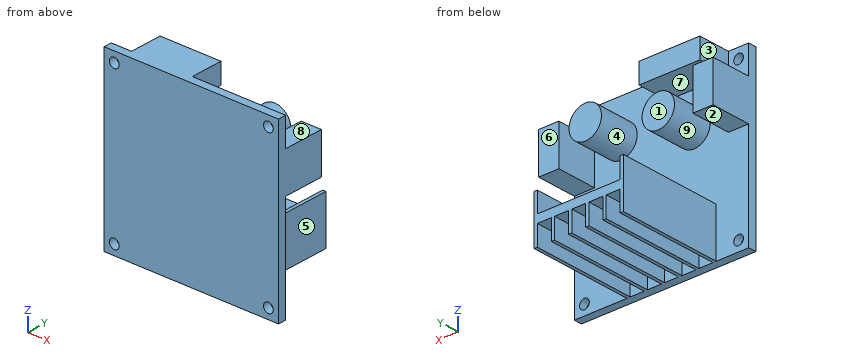
from build123d import *

# Parameters (mm, degrees)
SKETCH_1_W          = 43
SKETCH_1_H          = 43
EXTRUDE_1_DEPTH     = 2
SKETCH_2_W          = 15
SKETCH_2_H          = 5
EXTRUDE_2_DEPTH     = 10
SKETCH_3_W          = 5
SKETCH_3_H          = 10
EXTRUDE_3_DEPTH     = 10
SKETCH_4_W          = 5
SKETCH_4_H          = 10
EXTRUDE_4_DEPTH     = 10
SKETCH_5_R          = 4
EXTRUDE_5_DEPTH     = 10
SKETCH_6_R          = 4
EXTRUDE_6_DEPTH     = 10
SKETCH_7_W          = 22
SKETCH_7_H          = 12
EXTRUDE_7_DEPTH     = 26
SKETCH_8_W          = 3.44
SKETCH_8_H          = 26
SKETCH_8_H_2        = 26.05521278
CUT_EXTRUDE_1_DEPTH = 5
SKETCH_11_W         = 20.4
SKETCH_11_H         = 26
CUT_EXTRUDE_2_DEPTH = 5
SKETCH_12_W         = 20.4
SKETCH_12_H         = 7.82225214
EXTRUDE_8_DEPTH     = 5
SKETCH_13_W         = 20.4
SKETCH_13_H         = 5.214716639
EXTRUDE_9_DEPTH     = 2
SKETCH_14_R         = 1.2
CUT_EXTRUDE_3_DEPTH = 2


with BuildPart() as part:
    # 草图1 → 凸台-拉伸1 (new body)
    with BuildSketch(Plane(origin=(0, 0, 0), x_dir=(1, 0, 0), z_dir=(0, 1, 0))):
        Rectangle(SKETCH_1_W, SKETCH_1_H)
    extrude(amount=EXTRUDE_1_DEPTH)

    # 草图2 → 凸台-拉伸2 (add)
    with BuildSketch(Plane(origin=(0, 0, 0), x_dir=(1, 0, 0), z_dir=(0, 1, 0))):
        with Locations((-9, -19)):
            Rectangle(SKETCH_2_W, SKETCH_2_H)
    extrude(amount=EXTRUDE_2_DEPTH)

    # 草图3 → 凸台-拉伸3 (add)
    with BuildSketch(Plane(origin=(0, 2, 0), x_dir=(1, 0, 0), z_dir=(0, 1, 0))):
        with Locations((-19, -9.5)):
            Rectangle(SKETCH_3_W, SKETCH_3_H)
    extrude(amount=EXTRUDE_3_DEPTH)

    # 草图4 → 凸台-拉伸4 (add)
    with BuildSketch(Plane(origin=(0, 2, 0), x_dir=(1, 0, 0), z_dir=(0, 1, 0))):
        with Locations((19, -9.5)):
            Rectangle(SKETCH_4_W, SKETCH_4_H)
    extrude(amount=EXTRUDE_4_DEPTH)

    # 草图5 → 凸台-拉伸5 (add)
    with BuildSketch(Plane(origin=(0, 2, 0), x_dir=(1, 0, 0), z_dir=(0, 1, 0))):
        with Locations((-8, -8)):
            Circle(SKETCH_5_R)
    extrude(amount=EXTRUDE_5_DEPTH)

    # 草图6 → 凸台-拉伸6 (add)
    with BuildSketch(Plane(origin=(0, 2, 0), x_dir=(1, 0, 0), z_dir=(0, 1, 0))):
        with Locations((10, -12)):
            Circle(SKETCH_6_R)
    extrude(amount=EXTRUDE_6_DEPTH)

    # 草图7 → 凸台-拉伸7 (add)
    with BuildSketch(Plane(origin=(0, 2, 0), x_dir=(1, 0, 0), z_dir=(0, 1, 0))):
        with Locations((-2.475742283, 15.5)):
            Rectangle(SKETCH_7_W, SKETCH_7_H)
    extrude(amount=EXTRUDE_7_DEPTH)

    # 草图8 → 切除-拉伸1 (cut)
    with BuildSketch(Plane(origin=(0, 0, -21.5), x_dir=(-1, 0, 0), z_dir=(0, 0, -1))):
        with Locations((10.955742283, 15)):
            Rectangle(SKETCH_8_W, SKETCH_8_H)
        with Locations((6.715742283, 14.97239361)):
            Rectangle(SKETCH_8_W, SKETCH_8_H_2)
        with Locations((2.475742283, 15)):
            Rectangle(SKETCH_8_W, SKETCH_8_H)
        with Locations((-1.764257717, 15)):
            Rectangle(SKETCH_8_W, SKETCH_8_H)
        with Locations((-6.004257717, 15)):
            Rectangle(SKETCH_8_W, SKETCH_8_H)
    extrude(amount=-CUT_EXTRUDE_1_DEPTH, mode=Mode.SUBTRACT)

    # 草图11 → 切除-拉伸2 (cut)
    with BuildSketch(Plane.XY.offset(-9.5)):
        with Locations((-2.475742283, 15)):
            Rectangle(SKETCH_11_W, SKETCH_11_H)
    extrude(amount=-CUT_EXTRUDE_2_DEPTH, mode=Mode.SUBTRACT)

    # 草图12 → 凸台-拉伸8 (add)
    with BuildSketch(Plane.XY.offset(-14.5)):
        with Locations((-2.475742283, 12.38380745)):
            Rectangle(SKETCH_12_W, SKETCH_12_H)
    extrude(amount=EXTRUDE_8_DEPTH)

    # 草图13 → 凸台-拉伸9 (add)
    with BuildSketch(Plane.XY.offset(-14.5)):
        with Locations((-2.475742283, 18.90229184)):
            Rectangle(SKETCH_13_W, SKETCH_13_H)
    extrude(amount=EXTRUDE_9_DEPTH)

    # 草图14 → 切除-拉伸3 (cut)
    with BuildSketch(Plane(origin=(0, 2, 0), x_dir=(1, 0, 0), z_dir=(0, 1, 0))):
        with Locations((-19, 19)):
            Circle(SKETCH_14_R)
        with Locations((19, 19)):
            Circle(SKETCH_14_R)
        with Locations((-19, -19)):
            Circle(SKETCH_14_R)
        with Locations((19, -19)):
            Circle(SKETCH_14_R)
    extrude(amount=-CUT_EXTRUDE_3_DEPTH, mode=Mode.SUBTRACT)


solid = part.part
The listing builds one solid part. Answer for the finished solid, in the listing's coordinates (mm). Face numbers are marked on the shaded views. A direction names the side the tool comes from. Round coordinates to 2 decimals unless told otherwise and drop trailing zeros. Write each loop counter-clockwise with the first axis right and the second up, starting at its lowest first coordinate (ties: lowest second). Pieces come first, ordered by that corner, then holes. Notation, with made-up numbers: M 4.25,63.5 L 54.25,63.5 A8 cw 54.25,70.5 Z; hole C 23,67 d9. An arc over 180 degrees is marked long. Write each question's results on one line, items separated by ' | '. Start each with the question number.
(1) The part is cut by section B-B, the plane x = -19. Write down the section's boundary in (y, z).
(2) The part is cut by section C-C, the plane y = 20.25. Write down the section's boundary in (x, z), and give its area (3 significant figures).
(3) The part is cut by section A-A, the plane z = 19. Write down the section's boundary in (x, y), and give its area (3 significant figures).
(4) Find the intervals of material crossed by line 1 (Z direction, x = -19, y = 1.5); line 2 (X direction, y = 16.5, z = -18.5), in increasing order.
(5) For the marked faces 1, 2, 3, 4 and 5, determine the directions among +Z, -Z, +X, -X, +Y, -Y from which every point of the face is accessible in a straight line to the end or side of a thin tool.
(6) The part is cut by section D-D, the plane z = 6. Write down the section's boundary in (x, y), and give its area (3 significant figures).
(7) Determine the mould class of the marked faces 6, 7, 8 and 9 for opening direction Z: +Z half, -Z half, draft (parallel to the pull), parting line (faces both ways), or undercut.
(8) Each of these flat-tipped pins is pushed along its axis until it touches: P1, Ø1.7, axis at x = 6, y = 10.5, coming from the -Z side; P2, Ø8, axis at x = 5.5, y = 8.5, coming from the +Z side; P3, Ø2.5, axis at x = -19.5, y = 6.5, coming from the +Z side; P4, Ø2, axis at y = 17, z = -7.5, coming from the +X side. Where does it stop, or does it pass through?
Worked answers:
1) outline: M 0,-21.5 L 2,-21.5 L 2,-20.2 L 0,-20.2 Z; M 0,-17.8 L 2,-17.8 L 2,4.5 L 12,4.5 L 12,14.5 L 2,14.5 L 2,17.8 L 0,17.8 Z; M 0,20.2 L 2,20.2 L 2,21.5 L 0,21.5 Z
2) outline: M -13.48,-21.5 L -12.68,-21.5 L -12.68,-16.5 L -9.24,-16.5 L -9.24,-21.5 L -8.44,-21.5 L -8.44,-16.5 L -5,-16.5 L -5,-21.5 L -4.2,-21.5 L -4.2,-16.5 L -0.76,-16.5 L -0.76,-21.5 L 0.04,-21.5 L 0.04,-16.5 L 3.48,-16.5 L 3.48,-21.5 L 4.28,-21.5 L 4.28,-16.5 L 7.72,-16.5 L 7.72,-21.5 L 8.52,-21.5 L 8.52,-9.5 L 7.72,-9.5 L 7.72,-12.5 L -12.68,-12.5 L -12.68,-9.5 L -13.48,-9.5 Z | area: 117 mm²
3) outline: M -21.5,0 L -20.2,0 L -20.2,2 L -21.5,2 Z; M -17.8,0 L 17.8,0 L 17.8,2 L -1.5,2 L -1.5,10 L -16.5,10 L -16.5,2 L -17.8,2 Z; M 20.2,0 L 21.5,0 L 21.5,2 L 20.2,2 Z | area: 196 mm²
4) line 1: z = -21.5 to -20.2, -17.8 to 17.8, 20.2 to 21.5 | line 2: x = -13.48 to -12.68, -9.24 to -8.44, -5 to -4.2, -0.76 to 0.04, 3.48 to 4.28, 7.72 to 8.52
5) face 1: +Z, +X, -X, +Y | face 2: -Z, -X, +Y | face 3: +Z, -X, +Y | face 4: +Y | face 5: -Z, +X, +Y
6) outline: M -21.5,0 L 21.5,0 L 21.5,12 L 16.5,12 L 16.5,2 L -4.54,2 L -4.54,12 L -11.46,12 L -11.46,2 L -16.5,2 L -16.5,12 L -21.5,12 Z | area: 255 mm²
7) face 6: draft | face 7: undercut | face 8: +Z half | face 9: undercut
8) P1: stops at z = -16.5 | P2: stops at z = 15.97 | P3: stops at z = 14.5 | P4: passes through
